from build123d import *

# Parameters (mm, degrees)
SKETCH1_R           = 55
BOSS_EXTRUDE1_DEPTH = 6
CUT_EXTRUDE1_DEPTH  = 4
SKETCH3_R           = 1.7
CUT_EXTRUDE2_DEPTH  = 7
CIRPATTERN1_COUNT   = 72
SKETCH4_R           = 4.25
CUT_EXTRUDE3_DEPTH  = 3
BOSS_EXTRUDE2_DEPTH = 6


with BuildPart() as part:
    # Sketch1 → Boss-Extrude1 (new body)
    with BuildSketch(Plane(origin=(0, 0, 0), x_dir=(1, 0, 0), z_dir=(0, 1, 0))):
        Circle(SKETCH1_R)
    extrude(amount=BOSS_EXTRUDE1_DEPTH)

    # Sketch2 → Cut-Extrude1 (cut)
    with BuildSketch(Plane(origin=(0, 6, 0), x_dir=(1, 0, 0), z_dir=(0, 1, 0))):
        Polygon((3.75277675, 6.5), (-3.75277675, 6.5), (-7.505553499, 0), (-3.75277675, -6.5), (3.75277675, -6.5), (7.505553499, 0), align=None)
    extrude(amount=-CUT_EXTRUDE1_DEPTH, mode=Mode.SUBTRACT)

    # Sketch3 → Cut-Extrude2 (cut, through all)
    with BuildSketch(Plane(origin=(0, 6, 0), x_dir=(1, 0, 0), z_dir=(0, 1, 0))):
        with Locations((0, 51)):
            Circle(SKETCH3_R)
    cut_extrude2 = extrude(amount=-CUT_EXTRUDE2_DEPTH, mode=Mode.SUBTRACT)

    # CirPattern1: Cut-Extrude2 ×72 about axis
    cirpattern1_axis = Axis((0, 0, 0), (0, 1, 0))
    for i in range(1, CIRPATTERN1_COUNT):
        add(cut_extrude2.rotate(cirpattern1_axis, i * 360 / CIRPATTERN1_COUNT), mode=Mode.SUBTRACT)

    # Sketch4 → Cut-Extrude3 (cut, through all)
    with BuildSketch(Plane(origin=(0, 2, 0), x_dir=(1, 0, 0), z_dir=(0, 1, 0))):
        Circle(SKETCH4_R)
    extrude(amount=-CUT_EXTRUDE3_DEPTH, mode=Mode.SUBTRACT)

    # Sketch5 → Boss-Extrude2 (add)
    with BuildSketch(Plane(origin=(0, 6, 0), x_dir=(1, 0, 0), z_dir=(0, 1, 0))):
        Polygon((-59.94315244, 2.5), (-65, 0), (-59.94315244, -2.5), (-54.94315244, -2.5), (-54.94315244, 2.5), align=None)
    extrude(amount=-BOSS_EXTRUDE2_DEPTH)


solid = part.part
Can you work these out from the model? Positions are in its coordinate system, mm. Coordinates: 2 decimals unless noted, no trailing zeros. Order: outer loops, then holes, each group sorted by start corner. A loop starts at its lowest first (then second) coordinate and runs counter-clockwise, first axis right, second up. Notation, with made-up numbers: (82, 4) - (140, 4) arc R29 ccw to (140, 27) - close; hole circle Ø10 at (-9.5, -17). An arc over 180 degrees is marked (long way). Answer as a JSON object with one key per item and string values. Group by question number.
Q1. Imagine slicing it at C-C (x = -25.5). Please give me the cut outline in (y, z), and give its area (3 significant figures).
Q2. Imagine slicing it at A-A (x = 0). Please give me the cut outline in (y, z).
Q3. Imagine slicing it at B-B (z = 13). Please give me the cut outline in (x, y).
Q4. We'd pull the mould along Z, two halves only. Please class faces 1 (the face through (-4.371, 3.042, 52.504)), 2 (the face through (-62.436, 3.042, -1.267)): +Z half, -Z half, draft (parallel to the pull), parting line (faces both ways), or undercut.
Q5. I need wall thicknesses on line 1 (X direction, y = 3.4, z = 18); line 2 (X direction, y = 3.5, z = 18.5); line 3 (Z direction, x = 47, y = 3.3). Which ranges of each line are inside material? Lowest first, please. Write a range as from..to.
Q6. Will these pins go through, and if not, where does the flat tip stop? P1, Ø3, axis at x = 50.81, z = 4.44, coming from the -Y side; P2, Ø1.5, axis at x = -27, y = 3, coming from the -Z side; P3, Ø2, axis at y = 1.5, z = -4, coming from the -X side; P4, Ø3, axis at x = 7, y = 2.5, coming from the +Z side.
Q7. Imagine slicing it at D-D (y = 1.1). Give the number of separate pieces and of enclosed holes in the cut face, and give its area (3 significant figures).
Determined:
{
 "1": {"outline": "(0, -48.73) - (6, -48.73) - (6, -45.87) - (0, -45.87) - close; (0, -42.47) - (6, -42.47) - (6, 42.47) - (0, 42.47) - close; (0, 45.87) - (6, 45.87) - (6, 48.73) - (0, 48.73) - close", "area": "544 mm2"},
 "2": {"outline": "(0, -55) - (6, -55) - (6, -52.7) - (0, -52.7) - close; (0, -49.3) - (6, -49.3) - (6, -6.5) - (2, -6.5) - (2, -4.25) - (0, -4.25) - close; (0, 4.25) - (2, 4.25) - (2, 6.5) - (6, 6.5) - (6, 49.3) - (0, 49.3) - close; (0, 52.7) - (6, 52.7) - (6, 55) - (0, 55) - close"},
 "3": {"outline": "(-53.44, 0) - (-50.95, 0) - (-50.95, 6) - (-53.44, 6) - close; (-47.57, 0) - (47.57, 0) - (47.57, 6) - (-47.57, 6) - close; (50.95, 0) - (53.44, 0) - (53.44, 6) - (50.95, 6) - close"},
 "4": {"face 1": "undercut", "face 2": "-Z half"},
 "5": {"line 1": "x = -51.97..-49.53, -46.32..46.32, 49.53..51.97", "line 2": "x = -51.8..-49.26, -46.59..46.59, 49.26..51.8", "line 3": "z = -28.57..-23.06, -20.04..-18.87, -16.02..16.02, 18.87..20.04, 23.06..28.57"},
 "6": {"P1": "passes through", "P2": "stops at z = -48.33", "P3": "stops at x = -54.92", "P4": "stops at z = 54.72"},
 "7": {"separate pieces": "1", "enclosed holes": "73", "area": "8,830 mm2"}
}
